from build123d import *

# Parameters (mm, degrees)
CROQUIS1_W              = 25
CROQUIS1_H              = 30
CROQUIS1_R              = 1.55
SALIENTE_EXTRUIR1_DEPTH = 23
CROQUIS2_W              = 9
CROQUIS2_H              = 16.632666969
CORTAR_EXTRUIR1_DEPTH   = 30
CROQUIS3_R              = 2.575
CORTAR_EXTRUIR2_DEPTH   = 25
CORTAR_EXTRUIR3_DEPTH   = 2.5
CROQUIS5_R              = 4.25
CORTAR_EXTRUIR4_DEPTH   = 4.5
CORTAR_EXTRUIR5_DEPTH   = 4.5
CORTAR_EXTRUIR6_DEPTH   = 25
REDONDEO2_R             = 1
REDONDEO3_R             = 1
REDONDEO4_R             = 5
CROQUIS8_R              = 2.575
CROQUIS8_R_2            = 2.05
SALIENTE_EXTRUIR2_DEPTH = 2.9
CORTAR_EXTRUIR7_DEPTH   = 1.5


with BuildPart() as part:
    # Croquis1 → Saliente-Extruir1 (new body)
    with BuildSketch(Plane(origin=(0, 0, 0), x_dir=(1, 0, 0), z_dir=(0, 1, 0))):
        with Locations((12.5, 15)):
            Rectangle(CROQUIS1_W, CROQUIS1_H)
        with Locations((12.5, 25)):
            Circle(CROQUIS1_R, mode=Mode.SUBTRACT)
        with Locations((12.5, 5)):
            Circle(CROQUIS1_R, mode=Mode.SUBTRACT)
    extrude(amount=SALIENTE_EXTRUIR1_DEPTH)

    # Croquis2 → Cortar-Extruir1 (cut)
    with BuildSketch(Plane(origin=(0, 0, -30), x_dir=(-1, 0, 0), z_dir=(0, 0, -1))):
        with Locations((-12.5, 14.683666516)):
            Rectangle(CROQUIS2_W, CROQUIS2_H)
    extrude(amount=-CORTAR_EXTRUIR1_DEPTH, mode=Mode.SUBTRACT)

    # Croquis3 → Cortar-Extruir2 (cut)
    with BuildSketch(Plane.ZY):
        with Locations((-15, 16.5)):
            Circle(CROQUIS3_R)
    extrude(amount=-CORTAR_EXTRUIR2_DEPTH, mode=Mode.SUBTRACT)

    # Croquis4 → Cortar-Extruir3 (cut)
    with BuildSketch(Plane.ZY):
        Polygon((-14.95180736, 20.541164535), (-18.475654829, 18.562318318), (-18.523847469, 14.521153783), (-15.04819264, 12.458835465), (-11.524345171, 14.437681682), (-11.476152531, 18.478846217), align=None)
    extrude(amount=-CORTAR_EXTRUIR3_DEPTH, mode=Mode.SUBTRACT)

    # Croquis5 → Cortar-Extruir4 (cut)
    with BuildSketch(Plane(origin=(25, 0, 0), x_dir=(0, 0, -1), z_dir=(1, 0, 0))):
        with Locations((15, 16.5)):
            Circle(CROQUIS5_R)
    extrude(amount=-CORTAR_EXTRUIR4_DEPTH, mode=Mode.SUBTRACT)

    # Croquis6 → Cortar-Extruir5 (cut)
    with BuildSketch(Plane(origin=(0, 6.367333031, 0), x_dir=(1, 0, 0), z_dir=(0, 1, 0))):
        Polygon((15.848631561, 25), (14.174315781, 27.9), (10.825684219, 27.9), (9.151368439, 25), (10.825684219, 22.1), (14.174315781, 22.1), align=None)
        Polygon((15.848631561, 5), (14.174315781, 7.9), (10.825684219, 7.9), (9.151368439, 5), (10.825684219, 2.1), (14.174315781, 2.1), align=None)
    extrude(amount=-CORTAR_EXTRUIR5_DEPTH, mode=Mode.SUBTRACT)

    # Croquis7 → Cortar-Extruir6 (cut)
    with BuildSketch(Plane.ZY):
        with BuildLine():
            Line((-22.745966692, 23), (-30, 23))
            Line((-30, 23), (-30, 8))
            ThreePointArc((-30, 8), (-27.536048339, 16.062460813), (-22.745966692, 23))
        make_face()
        with BuildLine():
            Line((0, 23), (-7.254033308, 23))
            ThreePointArc((-7.254033308, 23), (-2.463951661, 16.062460813), (0, 8))
            Line((0, 8), (0, 23))
        make_face()
    extrude(amount=-CORTAR_EXTRUIR6_DEPTH, mode=Mode.SUBTRACT)

    # Redondeo2
    redondeo2_edges = [part.edges().sort_by_distance(p)[0] for p in [
        (8, 6.367333031, -15),
        (17, 6.367333031, -15),
    ]]
    fillet(redondeo2_edges, radius=REDONDEO2_R)

    # Redondeo3
    redondeo3_edges = [part.edges().sort_by_distance(p)[0] for p in [
        (25, 4, -30),
        (0, 4, -30),
        (25, 4, 0),
        (0, 4, 0),
    ]]
    fillet(redondeo3_edges, radius=REDONDEO3_R)

    # Redondeo4
    redondeo4_edges = [part.edges().sort_by_distance(p)[0] for p in [
        (4, 23, -22.745966692),
        (21, 23, -22.745966692),
        (4, 23, -7.254033308),
        (21, 23, -7.254033308),
    ]]
    fillet(redondeo4_edges, radius=REDONDEO4_R)

    # Croquis8 → Saliente-Extruir2 (add)
    with BuildSketch(Plane.ZY.offset(-2.5)):
        with Locations((-15, 16.5)):
            Circle(CROQUIS8_R)
        with Locations((-15, 16.5)):
            Circle(CROQUIS8_R_2, mode=Mode.SUBTRACT)
    extrude(amount=-SALIENTE_EXTRUIR2_DEPTH)

    # Croquis9 → Cortar-Extruir7 (cut)
    with BuildSketch(Plane.ZY.offset(-2.5)):
        Polygon((-11.476152531, 18.478846217), (-14.95180736, 20.541164535), (-18.475654829, 18.562318318), (-18.523847469, 14.521153783), (-15.04819264, 12.458835465), (-11.524345171, 14.437681682), align=None)
    extrude(amount=-CORTAR_EXTRUIR7_DEPTH, mode=Mode.SUBTRACT)


solid = part.part
The model under review builds one solid part; all positions refer to its coordinate system, in mm. A direction names the side the tool comes from. Coordinates: 2 decimals unless noted, no trailing zeros. Write each loop counter-clockwise with the first axis right and the second up, starting at its lowest first coordinate (ties: lowest second). Pieces come first, ordered by that corner, then holes. Notation, with made-up numbers: (15.25, -38) - (44.25, -38) arc R22 cw to (44.25, -27) - close; hole circle Ø9 at (-16.75, 34.25). An arc over 180 degrees is marked (long way). Answer as a JSON object with one key per item and string values. Group by question number.
1. Mouldability with a two-part tool opening along Y and no side actions: class faces 4 (the face through (6.682, 16.613, -17.573)), 5 (the face through (0, 11, -15)), 6 (the face through (16.715, 6.668, -14.79)), 7 (the face through (2, 19.5, -13.2)) as pulls with the +Y half, pulls with the -Y half, needs draft (parallel to the pull), parting line crosses it, or undercut.
2. Add section C-C (z = -6). Give the boundary of the cut face in (x, y).
3. Machinability: for faces 1 (the face through (13, 6.367, -15)), 2 (the face through (3.94, 14.82, -28.1)), 3 (the face through (13, 4, -7.9)), which of the approach directions +Z, -Z, +X, -X, +Y, -Y give a long, thin tool a straight path to every point of the face, cutting with its end or side? Answer none if there is none.
4. Clearance check with flat-ended pins moving along their axes: pin 1 Ø7 at (y, z) = (17.5, -17) entering from +X; pin 2 Ø3.5 at (x, z) = (12.5, -5) entering from +Y; pin 3 Ø2.5 at (y, z) = (15.5, -15) entering from +X; pin 4 Ø6 at (x, y) = (7, 16) entering from +Z. State where each tip first meets the part, or that it passes through.
5. Add section B-B (y = 16). Give the boundary of the cut face in (x, z).
6. Add section D-D (x = 12.5). Give the boundary of the cut face in (y, z).
7. To check wall thickness, follow probe 1 along X at (y, z) = (17.75, -10); probe 2 along Z at (x, y) = (12.5, 1.2); probe 3 along X at (y, z) = (1.1, -25). State the ranges of each line that lie inside material, in increasing order.
8. Add section A-A (x = 18.25). Give the boundary of the cut face in (y, z) (3 decimals), plus the area to 3 significant figures.
Findings:
{
 "1": {"face 4": "undercut", "face 5": "needs draft", "face 6": "pulls with the +Y half", "face 7": "undercut"},
 "2": {"outline": "(0, 0) - (11.32, 0) - (11.32, 1.87) - (9.73, 1.87) - (9.73, 6.37) - (9, 6.37) arc R1 cw to (8, 7.37) - (8, 21.54) - (0, 21.54) - close; (13.68, 0) - (25, 0) - (25, 21.54) - (17, 21.54) - (17, 7.37) arc R1 cw to (16, 6.37) - (15.27, 6.37) - (15.27, 1.87) - (13.68, 1.87) - close"},
 "3": {"face 1": "+Z, -Z, +Y", "face 2": "-Z, +X, -X, +Y", "face 3": "+Y"},
 "4": {"pin 1": "x = 25", "pin 2": "y = 1.87", "pin 3": "x = 5.4", "pin 4": "z = -1.2"},
 "5": {"outline": "(0, -27.57) - (8, -27.57) - (8, -17.53) - (5.4, -17.53) - (5.4, -16.99) - (4, -16.99) - (4, -18.51) - (0, -18.51) - close; (0, -11.51) - (4, -11.51) - (4, -13.01) - (5.4, -13.01) - (5.4, -12.47) - (8, -12.47) - (8, -2.43) - (0, -2.43) - close; (17, -27.57) - (25, -27.57) - (25, -19.22) - (20.5, -19.22) - (20.5, -17.53) - (17, -17.53) - close; (17, -12.47) - (20.5, -12.47) - (20.5, -10.78) - (25, -10.78) - (25, -2.43) - (17, -2.43) - close"},
 "6": {"outline": "(0, -30) - (6.37, -30) - (6.37, -27.9) - (1.87, -27.9) - (1.87, -26.55) - (0, -26.55) - close; (0, -23.45) - (1.87, -23.45) - (1.87, -22.1) - (6.37, -22.1) - (6.37, -7.9) - (1.87, -7.9) - (1.87, -6.55) - (0, -6.55) - close; (0, -3.45) - (1.87, -3.45) - (1.87, -2.1) - (6.37, -2.1) - (6.37, 0) - (0, 0) - close"},
 "7": {"probe 1": "0 to 8, 17 to 25", "probe 2": "-30 to -26.55, -23.45 to -6.55, -3.45 to 0", "probe 3": "0 to 10.95, 14.05 to 25"},
 "8": {"outline": "(0, -30) - (8, -30) arc R27.507 ccw to (21.091, -24.395) arc R5 ccw to (23, -20.464) - (23, -9.536) arc R5 ccw to (21.091, -5.605) arc R27.507 ccw to (8, 0) - (0, 0) - close; hole circle Ø5.15 at (16.5, -15)", "area": "588 mm²"}
}
